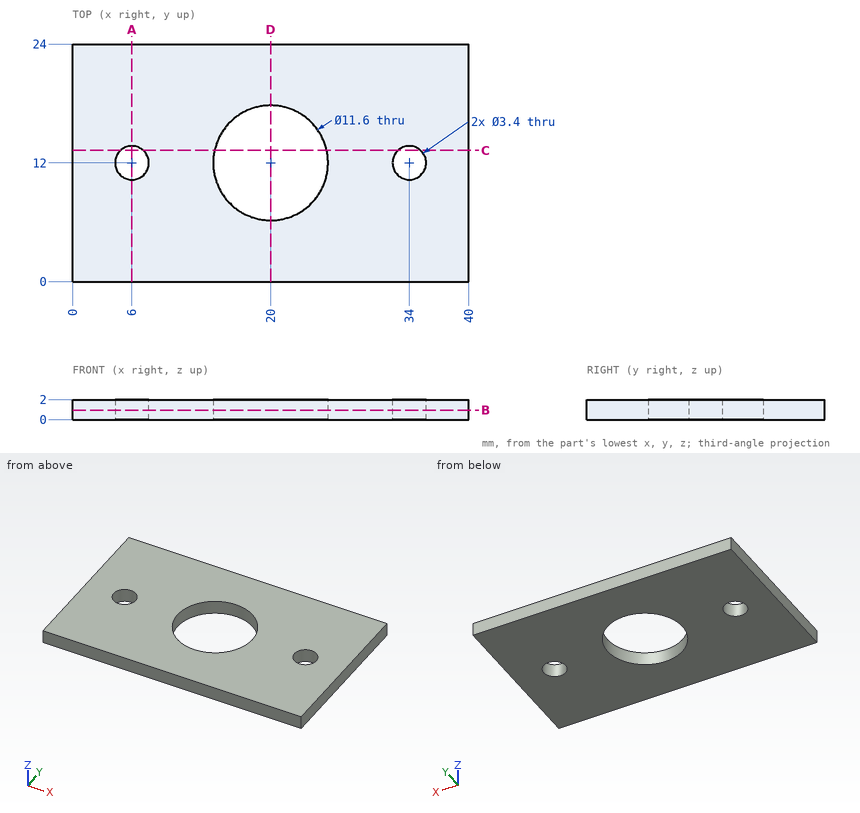
The figure shows three views and two pictorial views of one solid part (mm, origin at its lowest corner). Answer the questions. Coordinates: 2 decimals unless noted, no trailing zeros. Loops run counter-clockwise (first coordinate to the right, second up) from the corner with the lowest first, then second, coordinate; pieces in that order, holes last.
1) Find the intervals of material crossed by L1, parallel to Y at x = 34, z = 1.35; L2, parallel to Y at x = 20, z = 1.4; L3, parallel to X at y = 11.5, z = 0.65, in increasing order.
2) Find section A-A on x = 6. Write down the section's boundary in (y, z).
3) Find section C-C on y = 13.25. Write down the section's boundary in (x, z).
4) Flat-ended cylindrical pins translate along their axes: pin 1 Ø3 at (x, y) = (6, 12) entering from +Z; pin 2 Ø4 at (x, y) = (34, 12) entering from +Z. Find the tip coordinate at first contact, or state that the pin passes through.
5) Find section B-B on z = 0.95. Write down the section's boundary in (x, y), then the cut area to 3 significant figures.
6) Find section D-D on x = 20. Write down the section's boundary in (y, z).
Values:
1. L1: y = 0 to 10.3, 13.7 to 24
1. L2: y = 0 to 6.2, 17.8 to 24
1. L3: x = 0 to 4.38, 7.62 to 14.22, 25.78 to 32.38, 35.62 to 40
2. outline: (0, 0) - (10.3, 0) - (10.3, 2) - (0, 2) - close; (13.7, 0) - (24, 0) - (24, 2) - (13.7, 2) - close
3. outline: (0, 0) - (4.85, 0) - (4.85, 2) - (0, 2) - close; (7.15, 0) - (14.34, 0) - (14.34, 2) - (7.15, 2) - close; (25.66, 0) - (32.85, 0) - (32.85, 2) - (25.66, 2) - close; (35.15, 0) - (40, 0) - (40, 2) - (35.15, 2) - close
4. pin 1: passes through
4. pin 2: stops at z = 2
5. outline: (0, 0) - (40, 0) - (40, 24) - (0, 24) - close; hole circle Ø3.4 at (6, 12); hole circle Ø11.6 at (20, 12); hole circle Ø3.4 at (34, 12)
5. area: 836 mm2
6. outline: (0, 0) - (6.2, 0) - (6.2, 2) - (0, 2) - close; (17.8, 0) - (24, 0) - (24, 2) - (17.8, 2) - close
